Source: CAD feature listing. Evaluate the final solid. Frame: model axes, mm. A direction names the side the tool comes from. Give positions to 0.01 mm unless a question says otherwise; leave off trailing zeros. Order: outer loops, then holes, each group sorted by start corner. A loop starts at its lowest first (then second) coordinate and runs counter-clockwise, first axis right, second up.
from build123d import *

# Parameters (mm, degrees)
BOSS_EXTRUDE1_DEPTH = 30.5
SKETCH4_W           = 24.2
SKETCH4_H           = 13
CUT_EXTRUDE2_DEPTH  = 25
CUT_EXTRUDE4_DEPTH  = 11.5
SKETCH7_W           = 31
SKETCH7_H           = 1.7
BOSS_EXTRUDE3_DEPTH = 7
BOSS_EXTRUDE4_DEPTH = 7
LPATTERN1_COUNT     = 8
LPATTERN1_PITCH     = 3.6
SKETCH11_W          = 12
SKETCH11_H          = 4.5
BOSS_EXTRUDE5_DEPTH = 3.5
FILLET1_R           = 2
FILLET2_R           = 2
FILLET5_R           = 3
SKETCH12_W          = 4
SKETCH12_H          = 3.5
SKETCH12_W_2        = 3.8
CUT_EXTRUDE5_DEPTH  = 12
FILLET6_R           = 1.5


with BuildPart() as part:
    # Sketch1 → Boss-Extrude1 (new body)
    with BuildSketch(Plane.XY):
        Polygon((0, 0), (0, -30), (12, -30), (12, -20), (5, 0), align=None)
    extrude(amount=-BOSS_EXTRUDE1_DEPTH)

    # Sketch4 → Cut-Extrude2 (cut)
    with BuildSketch(Plane.ZY):
        with Locations((-14.4, -25.899949695)):
            Rectangle(SKETCH4_W, SKETCH4_H)
    extrude(amount=-CUT_EXTRUDE2_DEPTH, mode=Mode.SUBTRACT)

    # Sketch6 → Cut-Extrude4 (cut, symmetric)
    with BuildSketch(Plane.XY.offset(-15.25)):
        Polygon((5, 0), (5, -14), (9.9, -14), align=None)
    extrude(amount=CUT_EXTRUDE4_DEPTH, both=True, mode=Mode.SUBTRACT)

    # Sketch7 → Boss-Extrude3 (add)
    with BuildSketch(Plane(origin=(0, -30, 0), x_dir=(1, 0, 0), z_dir=(0, 1, 0))):
        with Locations((-4.2231607, 25.9)):
            Rectangle(SKETCH7_W, SKETCH7_H)
    extrude(amount=BOSS_EXTRUDE3_DEPTH)

    # Sketch10 → Boss-Extrude4 (add)
    with BuildSketch(Plane(origin=(0, -30, 0), x_dir=(1, 0, 0), z_dir=(0, 1, 0))):
        with BuildLine():
            Line((10.621636646, 22.381188189), (9.701086249, 22.381188189))
            ThreePointArc((9.701086249, 22.381188189), (9.246170102, 23.293637842), (9.190157183, 24.311663197))
            ThreePointArc((9.190157183, 24.311663197), (9.009091816, 24.685106498), (8.811361447, 25.05))
            Line((8.811361447, 25.05), (11.511361447, 25.05))
            ThreePointArc((11.511361447, 25.05), (11.313631078, 24.685106498), (11.132565711, 24.311663197))
            ThreePointArc((11.132565711, 24.311663197), (11.076552792, 23.293637842), (10.621636646, 22.381188189))
        make_face()
    boss_extrude4 = extrude(amount=BOSS_EXTRUDE4_DEPTH)

    # LPattern1: Boss-Extrude4 ×8
    with Locations(*[(-i * LPATTERN1_PITCH, 0, 0) for i in range(1, LPATTERN1_COUNT)]):
        add(boss_extrude4)

    # Sketch11 → Boss-Extrude5 (add)
    with BuildSketch(Plane(origin=(0, 0, -30.5), x_dir=(-1, 0, 0), z_dir=(0, 0, -1))):
        with Locations((-6, -27.75)):
            Rectangle(SKETCH11_W, SKETCH11_H)
    boss_extrude5 = extrude(amount=BOSS_EXTRUDE5_DEPTH)

    # Fillet1
    fillet1_edges = [part.edges().sort_by_distance(p)[0] for p in [
        (6, -25.5, -34),
    ]]
    fillet(fillet1_edges, radius=FILLET1_R)

    # Mirror1: Boss-Extrude5 across plane
    add(boss_extrude5.mirror(Plane.XY.offset(-15.25)))

    # Fillet2
    fillet2_edges = [part.edges().sort_by_distance(p)[0] for p in [
        (6, -25.5, 3.5),
    ]]
    fillet(fillet2_edges, radius=FILLET2_R)

    # Fillet5
    fillet5_edges = [part.edges().sort_by_distance(p)[0] for p in [
        (5, -14, -15.25),
        (5.894991197, -19.399949695, -2.3),
        (5.894991197, -19.399949695, -26.5),
    ]]
    fillet(fillet5_edges, radius=FILLET5_R)

    # Sketch12 → Cut-Extrude5 (cut)
    with BuildSketch(Plane.ZY):
        with Locations((-30.494628275, -28.768411502)):
            Rectangle(SKETCH12_W, SKETCH12_H)
        with Locations((0.6, -28.814354386)):
            Rectangle(SKETCH12_W_2, SKETCH12_H)
    extrude(amount=-CUT_EXTRUDE5_DEPTH, mode=Mode.SUBTRACT)

    # Fillet6
    fillet6_edges = [part.edges().sort_by_distance(p)[0] for p in [
        (6, -27.018411502, -28.494628275),
        (6, -27.018411502, -32.494628275),
        (6, -27.064354386, -1.3),
        (6, -27.064354386, 2.5),
    ]]
    fillet(fillet6_edges, radius=FILLET6_R)


solid = part.part
1) Section query C-C on z = -27.5. Output: boundary loops of the cut face in (x, y), and give its area (3 significant figures).
Checks:
outline: (0, -30) - (12, -30) - (12, -20) - (5, 0) - (0, 0) - close
area: 290 mm2
2) Section query B-B on z = -15.5. Output: boundary loops of the cut face in (x, y), and give its area (3 significant figures).
Checks:
outline: (0, -19.4) - (11.79, -19.4) - (9.9, -14) - (8, -14) arc R3 cw to (5, -11) - (5, 0) - (0, 0) - close
area: 130 mm2
3) Section query D-D on y = -16.25. Output: boundary loops of the cut face in (x, z), and give its area (3 significant figures).
Checks:
outline: (0, -30.5) - (10.69, -30.5) - (10.69, 0) - (0, 0) - close
area: 326 mm2
4) Ray query, L1, parallel to X at y = -8.25, z = -25; L2, parallel to Y at x = 6, z = -24.5; L3, parallel to Z at x = 5, y = -19.25. Return the intervals inside material, ascending.
Checks:
L1: x = 0 to 5
L2: y = -30 to -23, -19.57 to -13.24
L3: z = -30.5 to 0
5) Pull-direction query (Y, two-part tool) for faces 1 (the face through (10.105, -14.584, -15.036)), 2 (the face through (-4, -23, -25)), 3 (the face through (-9.6, -26.5, -25.05)), 4 (the face through (6, -30, 3)); classes: +Y half, -Y half, draft (parallel to the pull), parting line (faces both ways), or undercut.
Checks:
face 1: +Y half
face 2: undercut
face 3: draft
face 4: -Y half
6) First-contact query: pin 1 Ø5 at (x, z) = (-0.5, -11.5) entering from -Y; pin 2 Ø1 at (y, z) = (-6, -6.5) entering from -X; pin 3 Ø0.5 at (x, y) = (1, -25) entering from +Z; pin 4 Ø10 at (x, z) = (-12.5, -16) entering from +Y. Flat tips, straight axial feed; report the tip coordinate or a pass-through.
Checks:
pin 1: stops at y = -19.4
pin 2: stops at x = 0
pin 3: stops at z = 0
pin 4: passes through
7) Section query A-A on y = -9. Output: boundary loops of the cut face in (x, z), and give its area (3 significant figures).
Checks:
outline: (0, -30.5) - (8.15, -30.5) - (8.15, -26.75) - (5, -26.75) - (5, -3.75) - (8.15, -3.75) - (8.15, 0) - (0, 0) - close
area: 176 mm2
8) Reachability of faces 5 (the face through (6, -29, -28.495)), 6 (the face through (-6.92, -26.55, -23.31)), 7 (the face through (5, -5, -15)), 8 (the face through (2.05, -26.55, -23.28)) from +Z, -Z, +X, -X, +Y, -Y: full face, straight path, thin tool, end or side. Return the list, or none.
Checks:
face 5: +X, -X, -Y
face 6: +Y, -Y
face 7: +X, +Y
face 8: -Y
